Autodesk Inventor part; units mm, degrees
ref_plane "YZ Plane" through (0, 0, 0) normal (1, 0, 0) x (0, 1, 0)
ref_plane "XZ Plane" through (0, 0, 0) normal (0, 1, 0) x (-1, 0, 0)
ref_plane "XY Plane" through (0, 0, 0) normal (0, 0, 1) x (1, 0, 0)
sketch "Sketch1" plane through (0, 0, 0) normal (0, 0, 1) x (1, 0, 0)
  circle A0 centre (0, 0) radius 2.95
  dimension "d0" = 5.9
extrude "Extrusion1" add sketch "Sketch1" along normal blind 4.5
sketch "Sketch2" plane through (0, 0, 0) normal (0, 0, -1) x (-1, 0, 0)
  circle A0 centre (0, 0) radius 4
  dimension "d3" = 8
extrude "Extrusion2" add sketch "Sketch2" along normal blind 11.7
sketch "Sketch3" plane through (0, 0, -11.7) normal (0, 0, -1) x (-1, 0, 0)
  line L0 (2.665, 1.1) -> (2.335, 1.1)
  line L1 (2.335, 1.1) -> (2.335, -1.1)
  line L2 (2.335, -1.1) -> (2.665, -1.1)
  line L3 (2.665, -1.1) -> (2.665, 1.1)
  line L4 (2.5, 1.1) -> (2.5, -1.1) construction
  line L5 (5.6, 0) -> (-5.6, 0) construction
  point P0 (0, 0)
  point P1 (2.5, 0)
  dimension "d6" = 0.33
  dimension "d7" = 2.2
  dimension "d8" = 2.5
extrude "Extrusion3" add sketch "Sketch3" along normal blind 6.3
sketch "Sketch4" plane through (0, 0, -11.7) normal (0, 0, -1) x (-1, 0, 0)
  line L0 (1, 2.65) -> (-1, 2.65)
  line L1 (-1, 2.65) -> (-1, 2.35)
  line L2 (-1, 2.35) -> (1, 2.35)
  line L3 (1, 2.35) -> (1, 2.65)
  line L4 (1, -2.35) -> (-1, -2.35)
  line L5 (-1, -2.35) -> (-1, -2.65)
  line L6 (-1, -2.65) -> (1, -2.65)
  line L7 (1, -2.65) -> (1, -2.35)
  line L8 (0, -5.6) -> (0, 5.6)
  line L9 (1, 2.5) -> (-1, 2.5) construction
  line L10 (-1, -2.5) -> (1, -2.5) construction
  line L11 (5.6, 0) -> (-5.6, 0) construction
  point P0 (0, 0)
  point P1 (0, 2.35)
  dimension "d11" = 2
  dimension "d12" = 0.3
  dimension "d13" = 5
extrude "Extrusion4" add sketch "Sketch4" along normal blind 3
properties part number "StereoBuchseEinbau"
Can you work these out from the model? Positions are in its coordinate system, mm. A direction names the side the tool comes from. Round coordinates to 2 decimals unless told otherwise and drop trailing zeros. Order: outer loops, then holes, each group sorted by start corner. A loop starts at its lowest first (then second) coordinate and runs counter-clockwise, first axis right, second up. Notation, with made-up numbers: (59, 88) -> (92, 88) arc R10 ccw to (92, 104) -> close; hole circle Ø8 at (56.5, 83). An arc over 180 degrees is marked (long way). Return JSON: item names as keys, results as strings. Group by question number.
1. If we section it at D-D, the plane x = -1.25: Write out the boundary of the cut face in (y, z).
2. I need wall thicknesses on line 1 (X direction, y = 0, z = -14.25) (3 decimals); line 2 (Z direction, x = -0.5, y = 3.5); line 3 (Z direction, x = 0, y = 0.5). Which ranges of each line are inside material? Lowest first, please. Write a range as [from, to].
3. If we section it at B-B, the plane y = 0: Write out the boundary of the cut face in (x, z) (3 decimals).
4. Will these pins go through, and if not, where does the flat tip stop? pin 1 (2.5 mm diameter, centred on y = 0, z = -16, fed in from +X) (3 decimals); pin 2 (1.5 mm diameter, centred on y = 2, z = -6.5, fed in from -X); pin 3 (2 mm diameter, centred on x = 0.5, z = -13.5, fed in from +Y).
5. We'd pull the mould along Y, two halves only. Please class faces 1 (the face through (0, 2.35, -13)), 2 (the face through (-2.665, 0, -15)), 3 (the face through (0.867, 3.905, -5.768)): released by +Y, released by -Y, zero draft, split by the parting line, or undercut.
6. Which directions (+Z, -Z, +X, -X, +Y, -Y) give clear straight access to the entire face, cutting with the end or side of a thin tool? Please do faces 4 (the face through (0, -2.35, -13)), 5 (the face through (0, -2.65, -13)), 6 (the face through (0, 2.65, -13)), 7 (the face through (-2.335, 0, -15)), 8 (the face through (2, -3, 0)).
7. If we section it at A-A, the plane x = 0: Write out the boundary of the cut face in (y, z), then the cut area to 3 significant figures.
8. If we section it at C-C, the plane z = -16: Write out the boundary of the cut face in (x, y) (3 decimals).
Output values:
{
 "1": {"outline": "(-3.8, -11.7) -> (3.8, -11.7) -> (3.8, 0) -> (2.67, 0) -> (2.67, 4.5) -> (-2.67, 4.5) -> (-2.67, 0) -> (-3.8, 0) -> close"},
 "2": {"line 1": "[-2.665, -2.335]", "line 2": "[-11.7, 0]", "line 3": "[-11.7, 4.5]"},
 "3": {"outline": "(-4, -11.7) -> (-2.665, -11.7) -> (-2.665, -18) -> (-2.335, -18) -> (-2.335, -11.7) -> (4, -11.7) -> (4, 0) -> (2.95, 0) -> (2.95, 4.5) -> (-2.95, 4.5) -> (-2.95, 0) -> (-4, 0) -> close"},
 "4": {"pin 1": "x = -2.335", "pin 2": "x = -3.8", "pin 3": "y = 2.65"},
 "5": {"face 1": "undercut", "face 2": "zero draft", "face 3": "split by the parting line"},
 "6": {"face 4": "-Z, +X, -X", "face 5": "-Z, +X, -X, -Y", "face 6": "-Z, +X, -X, +Y", "face 7": "-Z, +X, +Y, -Y", "face 8": "+Z"},
 "7": {"outline": "(-4, -11.7) -> (-2.65, -11.7) -> (-2.65, -14.7) -> (-2.35, -14.7) -> (-2.35, -11.7) -> (2.35, -11.7) -> (2.35, -14.7) -> (2.65, -14.7) -> (2.65, -11.7) -> (4, -11.7) -> (4, 0) -> (2.95, 0) -> (2.95, 4.5) -> (-2.95, 4.5) -> (-2.95, 0) -> (-4, 0) -> close", "area": "122 mm²"},
 "8": {"outline": "(-2.665, -1.1) -> (-2.335, -1.1) -> (-2.335, 1.1) -> (-2.665, 1.1) -> close"}
}
